```python
from build123d import *

# Parameters (mm, degrees)
ESBO_O1_W                = 143.01
ESBO_O1_H                = 54.05
RESSALTO_EXTRUS_O1_DEPTH = 6.35
ESBO_O2_R                = 2.755
ESBO_O2_R_2              = 2.755565393
ESBO_O2_R_3              = 2.735691737
CORTE_EXTRUS_O1_DEPTH    = 6.35
ESBO_O3_R                = 15.995
ESBO_O3_R_2              = 10
CORTE_EXTRUS_O2_DEPTH    = 10
ESBO_O4_W                = 143.01
ESBO_O4_H                = 3.42
RESSALTO_EXTRUS_O2_DEPTH = 6.35
ESBO_O5_R                = 16
CORTE_EXTRUS_O3_DEPTH    = 10
CROQUIS1_W               = 143.01
CROQUIS1_H               = 2
SALIENTE_EXTRUIR2_DEPTH  = 6.35
ESBO_O6_R                = 1.5
CORTE_EXTRUS_O4_DEPTH    = 17


with BuildPart() as part:
    # Esboço1 → Ressalto-extrusão1 (new body)
    with BuildSketch(Plane.XY):
        Rectangle(ESBO_O1_W, ESBO_O1_H)
    extrude(amount=RESSALTO_EXTRUS_O1_DEPTH)

    # Esboço2 → Corte-extrusão1 (cut)
    with BuildSketch(Plane(origin=(0, 0, 0), x_dir=(-1, 0, 0), z_dir=(0, 0, -1))):
        with Locations((-44.463136928, 23.291850449)):
            Circle(ESBO_O2_R)
        with Locations((-65.913136928, 1.841850449)):
            Circle(ESBO_O2_R_2)
        with Locations((-44.463136928, -19.608149551)):
            Circle(ESBO_O2_R_3)
        with Locations((-23.013136928, 1.841850449)):
            Circle(ESBO_O2_R)
        with Locations((23.016863072, 1.841850449)):
            Circle(ESBO_O2_R)
        with Locations((44.466863072, -19.608149551)):
            Circle(ESBO_O2_R)
        with Locations((65.916863072, 1.841850449)):
            Circle(ESBO_O2_R)
        with Locations((44.466863072, 23.291850449)):
            Circle(ESBO_O2_R)
    extrude(amount=-CORTE_EXTRUS_O1_DEPTH, mode=Mode.SUBTRACT)

    # Esboço3 → Corte-extrusão2 (cut)
    with BuildSketch(Plane(origin=(0, 0, 0), x_dir=(-1, 0, 0), z_dir=(0, 0, -1))):
        with Locations((-44.463136928, 1.841850449)):
            Circle(ESBO_O3_R)
        with Locations((0.001863072, 1.841850449)):
            Circle(ESBO_O3_R_2)
        with Locations((44.466863072, 1.841850449)):
            Circle(ESBO_O3_R)
    extrude(amount=-CORTE_EXTRUS_O2_DEPTH, mode=Mode.SUBTRACT)

    # Esboço4 → Ressalto-extrusão2 (add)
    with BuildSketch(Plane.XY):
        with Locations((0, 28.735)):
            Rectangle(ESBO_O4_W, ESBO_O4_H)
    extrude(amount=RESSALTO_EXTRUS_O2_DEPTH)

    # Esboço5 → Corte-extrusão3 (cut)
    with BuildSketch(Plane.XY.offset(6.35)):
        with Locations((-0.001863072, 1.841850449)):
            Circle(ESBO_O5_R)
    extrude(amount=-CORTE_EXTRUS_O3_DEPTH, mode=Mode.SUBTRACT)

    # Croquis1 → Saliente-Extruir2 (add)
    with BuildSketch(Plane.XY.offset(6.35)):
        with Locations((0, 31.445)):
            Rectangle(CROQUIS1_W, CROQUIS1_H)
    extrude(amount=-SALIENTE_EXTRUIR2_DEPTH)

    # Esboço6 → Corte-extrusão4 (cut)
    with BuildSketch(Plane(origin=(0, 32.445, 0), x_dir=(1, 0, 0), z_dir=(0, 1, 0))):
        with Locations(Location((56.423186497, -3.175, 0), (0, 0, 270))):
            Circle(ESBO_O6_R)
        with Locations(Location((26.423186497, -3.175, 0), (0, 0, 270))):
            Circle(ESBO_O6_R)
        with Locations(Location((-26.423186497, -3.175, 0), (0, 0, 90))):
            Circle(ESBO_O6_R)
        with Locations(Location((-56.423186497, -3.175, 0), (0, 0, 90))):
            Circle(ESBO_O6_R)
    extrude(amount=-CORTE_EXTRUS_O4_DEPTH, mode=Mode.SUBTRACT)


solid = part.part
```
Part model, mm, in its own coordinate system. A direction names the side the tool comes from. Round coordinates to 2 decimals unless told otherwise and drop trailing zeros. Loops run counter-clockwise (first coordinate to the right, second up) from the corner with the lowest first, then second, coordinate; pieces in that order, holes last.
Item 1: Mould opens along Z. For faces 1 (the face through (-17, 3, 0)), 2 (the face through (-54.96, 24.06, 3.5)), 3 (the face through (-42.281, 21.615, 3.131)), 4 (the face through (-56, 15.445, 3)) say: +Z half, -Z half, draft (parallel to the pull), parting line (faces both ways), or undercut.
Item 2: 3-axis set-ups, long thin cutter, end or side, ignore diameter. For faces 5 (the face through (67.944, 3.704, 3.131)), 6 (the face through (27.69, 24.06, 3.98)): which of +Z, -Z, +X, -X, +Y, -Y reach the whole face in a straight line?
Item 3: Cut at B-B, the plane y = -5. State how many separate pieces and enclosed holes the cut face has, then the cut area to 3 significant figures.
Item 4: Cut at A-A, the plane x = -36.5. Give the cut face in (y, z) (3 decimals), then the cut area to 3 significant figures.
Item 5: Drop a flat-ended pin along its axis: P1, Ø2.5, axis at x = 26.42, z = 3.18, coming from the +Y side (3 decimals). Give the stop position or say it passes through.
Item 6: Drill centre lines: line 1 (X direction, y = 10, z = 0.5) (3 decimals); line 2 (X direction, y = 13.5, z = 5) (3 decimals); line 3 (Y direction, x = -39.5, z = 2) (3 decimals). Where is each one in solid material? Low to high.
Item 7: Cut at D-D, the plane y = 11. Give the cut face in (x, z) (3 decimals).
A:
1. face 1: -Z half
1. face 2: undercut
1. face 3: draft
1. face 4: undercut
2. face 5: +Z, -Z
2. face 6: +Y
3. separate pieces: 4
3. enclosed holes: 0
3. area: 357 mm2
4. outline: (-27.025, 0) - (-12.028, 0) - (-12.028, 6.35) - (-27.025, 6.35) - close; (15.712, 0) - (32.445, 0) - (32.445, 6.35) - (15.712, 6.35) - close
4. area: 201 mm2
5. P1: stops at y = 15.445
6. line 1: x = -71.505 to -58.225, -30.709 to -13.766, 13.762 to 30.705, 58.221 to 71.505
6. line 2: x = -71.505 to -55.418, -33.516 to -10.96, 10.957 to 33.512, 55.414 to 71.505
6. line 3: y = -27.025 to -13.362, 17.046 to 32.445
7. outline: (-71.505, 0) - (-57.581, 0) - (-57.581, 6.35) - (-71.505, 6.35) - close; (-31.353, 0) - (-13.122, 0) - (-13.122, 6.35) - (-31.353, 6.35) - close; (13.118, 0) - (31.349, 0) - (31.349, 6.35) - (13.118, 6.35) - close; (57.577, 0) - (71.505, 0) - (71.505, 6.35) - (57.577, 6.35) - close
